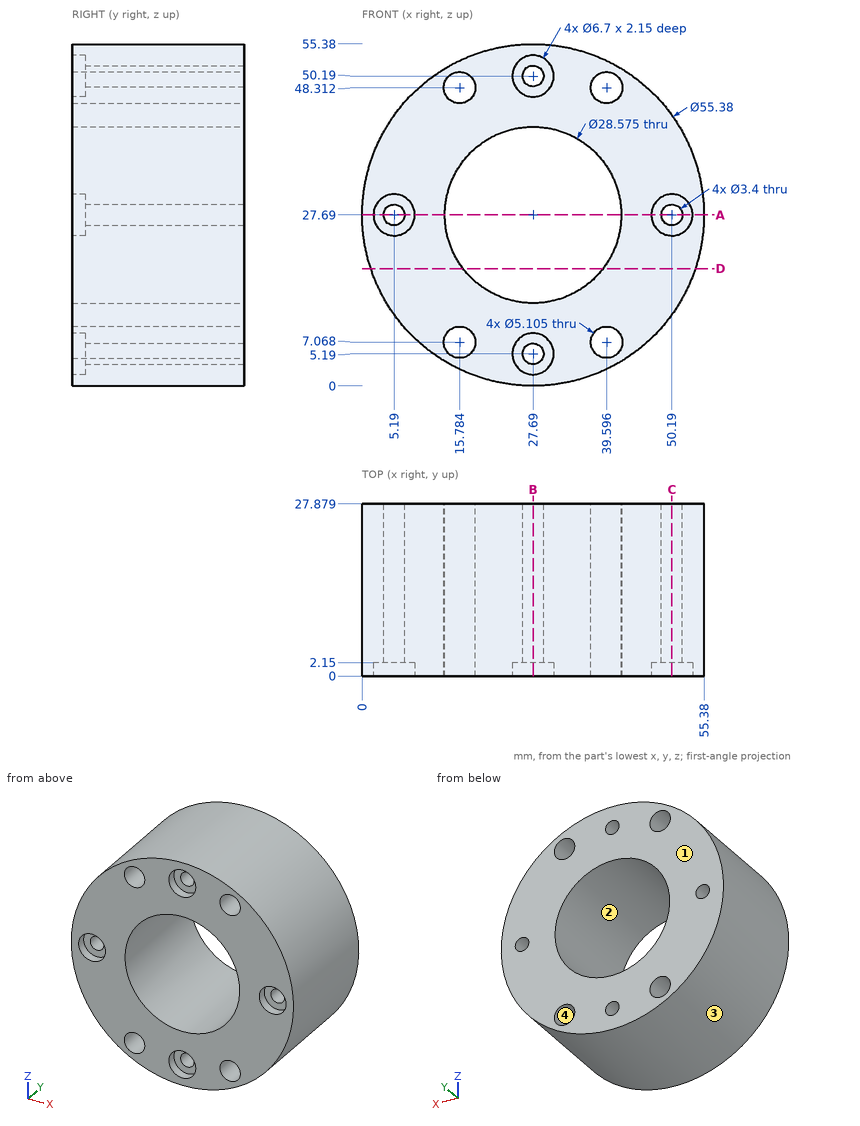
Can you work these out from the drawing? Everything is in mm from the part's minimum corner. Round coordinates to 2 decimals unless told otherwise and drop trailing zeros. Order: outer loops, then holes, each group sorted by start corner. A loop starts at its lowest first (then second) coordinate and runs counter-clockwise, first axis right, second up. Notation, with made-up numbers: (-23.75, 24) -> (1.25, 24) arc R28 ccw to (1.25, 47) -> close; hole circle Ø3 at (36, -13.75). An arc over 180 degrees is marked (long way). Return JSON: item names as keys, results as strings. Group by question number.
1. If we section it at A-A, the plane z = 27.69: Write out the boundary of the cut face in (x, y).
2. Will these pins go through, and if not, where does the flat tip stop? pin 1 (3.5 mm diameter, centred on x = 28.5, z = 49, fed in from -Y); pin 2 (12 mm diameter, centred on x = 14, y = 12, fed in from -Z); pin 3 (12 mm diameter, centred on x = 12, y = 15, fed in from -Z).
3. We'd pull the mould along X, two halves only. Please class the marked faces 1, 2, 3 and 4: released by +X, released by -X, zero draft, split by the parting line, or undercut.
4. If we section it at C-C, the plane x = 50.19: Write out the boundary of the cut face in (y, z).
5. If we section it at D-D, the plane z = 19: Write out the boundary of the cut face in (x, y).
6. If we section it at B-B, the plane x = 27.69: Write out the boundary of the cut face in (y, z).
7. I need wall thicknesses on line 1 (X direction, y = 18.75, z = 47) (1 decimal); line 2 (Z direction, x = 50, y = 21.25); line 3 (Y direction, x = 5.5, z = 25). Which ranges of each line are inside material? Lowest first, please. Write a range as [from, to].
Output values:
{
 "1": {"outline": "(0, 0) -> (1.84, 0) -> (1.84, 2.15) -> (3.49, 2.15) -> (3.49, 27.88) -> (0, 27.88) -> close; (6.89, 2.15) -> (8.54, 2.15) -> (8.54, 0) -> (13.4, 0) -> (13.4, 27.88) -> (6.89, 27.88) -> close; (41.98, 0) -> (46.84, 0) -> (46.84, 2.15) -> (48.49, 2.15) -> (48.49, 27.88) -> (41.98, 27.88) -> close; (51.89, 2.15) -> (53.54, 2.15) -> (53.54, 0) -> (55.38, 0) -> (55.38, 27.88) -> (51.89, 27.88) -> close"},
 "2": {"pin 1": "y = 2.15", "pin 2": "z = 1.09", "pin 3": "z = 1.75"},
 "3": {"face 1": "zero draft", "face 2": "undercut", "face 3": "split by the parting line", "face 4": "undercut"},
 "4": {"outline": "(0, 11.55) -> (27.88, 11.55) -> (27.88, 25.99) -> (2.15, 25.99) -> (2.15, 24.34) -> (0, 24.34) -> close; (0, 31.04) -> (2.15, 31.04) -> (2.15, 29.39) -> (27.88, 29.39) -> (27.88, 43.83) -> (0, 43.83) -> close"},
 "5": {"outline": "(1.4, 0) -> (16.35, 0) -> (16.35, 27.88) -> (1.4, 27.88) -> close; (39.03, 0) -> (53.98, 0) -> (53.98, 27.88) -> (39.03, 27.88) -> close"},
 "6": {"outline": "(0, 0) -> (27.88, 0) -> (27.88, 3.49) -> (2.15, 3.49) -> (2.15, 1.84) -> (0, 1.84) -> close; (0, 8.54) -> (2.15, 8.54) -> (2.15, 6.89) -> (27.88, 6.89) -> (27.88, 13.4) -> (0, 13.4) -> close; (0, 41.98) -> (27.88, 41.98) -> (27.88, 48.49) -> (2.15, 48.49) -> (2.15, 46.84) -> (0, 46.84) -> close; (0, 53.54) -> (2.15, 53.54) -> (2.15, 51.89) -> (27.88, 51.89) -> (27.88, 55.38) -> (0, 55.38) -> close"},
 "7": {"line 1": "[7.8, 13.6], [18, 37.4], [41.8, 47.5]", "line 2": "[11.29, 26], [29.38, 44.09]", "line 3": "[2.15, 27.88]"}
}
